Check sheet for the modelled part. Datum: model origin and axes. Units: mm. Face numbers are marked on the shaded views. Round coordinates to 2 decimals unless told otherwise and drop trailing zeros. Write each loop counter-clockwise with the first axis right and the second up, starting at its lowest first coordinate (ties: lowest second). Pieces come first, ordered by that corner, then holes. Notation, with made-up numbers: M 68,80 L 114,80 A22 ccw 114,91 Z; hole C 13.25,76.25 d9. An arc over 180 degrees is marked long. Put each result on its own line as item: value.
```python
from build123d import *

# Parameters (mm, degrees)
SKETCH1_W           = 117
SKETCH1_H           = 133.1
SKETCH1_R           = 2.75
SKETCH1_R_2         = 3.38
SKETCH1_R_3         = 12.5
BOSS_EXTRUDE1_DEPTH = 6.35


with BuildPart() as part:
    # Sketch1 → Boss-Extrude1 (new body)
    with BuildSketch(Plane.XY):
        with Locations((0, 3.45)):
            Rectangle(SKETCH1_W, SKETCH1_H)
        with Locations((-48.75, -18.4)):
            Circle(SKETCH1_R, mode=Mode.SUBTRACT)
        with Locations((48.75, -18.4)):
            Circle(SKETCH1_R, mode=Mode.SUBTRACT)
        with Locations((-10.368974359, 60.010374765)):
            Circle(SKETCH1_R, mode=Mode.SUBTRACT)
        with Locations((-40, -44.05)):
            Circle(SKETCH1_R_2, mode=Mode.SUBTRACT)
        with Locations((40, -44.05)):
            Circle(SKETCH1_R_2, mode=Mode.SUBTRACT)
        Circle(SKETCH1_R_3, mode=Mode.SUBTRACT)
    extrude(amount=BOSS_EXTRUDE1_DEPTH)


solid = part.part
```
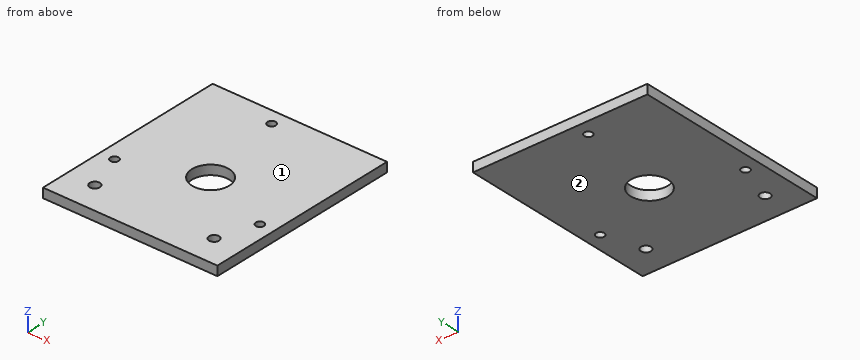
1. Scan lines: probe 1 along X at (y, z) = (-44, 2); probe 2 along Y at (x, z) = (0, 2.75); probe 3 along Y at (x, z) = (-48.75, 3.5). Record each from-to range of solid material in increasing order.
Computed values:
probe 1: x = -58.5 to -43.38, -36.62 to 36.62, 43.38 to 58.5
probe 2: y = -63.1 to -12.5, 12.5 to 70
probe 3: y = -63.1 to -21.15, -15.65 to 70
2. Release check for a two-part mould opening along Z. For the marked faces 1 and 2 record: +Z half, -Z half, draft (parallel to the pull), parting line (faces both ways), or undercut.
Computed values:
face 1: +Z half
face 2: -Z half
3. Cross-section at D-D (y = 0). Enter the section's corners in (x, z), then the cut area to 3 significant figures.
Computed values:
outline: M -58.5,0 L -12.5,0 L -12.5,6.35 L -58.5,6.35 Z; M 12.5,0 L 58.5,0 L 58.5,6.35 L 12.5,6.35 Z
area: 584 mm2
4. Cross-section at A-A (x = -40). Enter the section's corners in (y, z).
Computed values:
outline: M -63.1,0 L -47.43,0 L -47.43,6.35 L -63.1,6.35 Z; M -40.67,0 L 70,0 L 70,6.35 L -40.67,6.35 Z
5. Cross-section at B-B (y = -18.4). Enter the section's corners in (x, z), then the cut area to 3 significant figures.
Computed values:
outline: M -58.5,0 L -51.5,0 L -51.5,6.35 L -58.5,6.35 Z; M -46,0 L 46,0 L 46,6.35 L -46,6.35 Z; M 51.5,0 L 58.5,0 L 58.5,6.35 L 51.5,6.35 Z
area: 673 mm2
6. Depth check by flat-ended pin: pin 1 Ø3.5 at (x, y) = (-10.37, 60.01) entering from +Z. Enter the tip coordinate at first touch or a pass-through.
Computed values:
pin 1: passes through
7. Cross-section at C-C (z = 2.25). Enter the section's corners in (x, y), then the cut area to 3 significant figures.
Computed values:
outline: M -58.5,-63.1 L 58.5,-63.1 L 58.5,70 L -58.5,70 Z; hole C -48.75,-18.4 d5.5; hole C -40,-44.05 d6.76; hole C -10.37,60.01 d5.5; hole C 0,0 d25; hole C 40,-44.05 d6.76; hole C 48.75,-18.4 d5.5
area: 14,900 mm2
